```python
from build123d import *

# Parameters (mm, degrees)
SKETCH_1_R          = 12.935
EXTRUDE_1_DEPTH     = 7
SKETCH_2_R          = 14.135
EXTRUDE_2_DEPTH     = 1
SKETCH_3_R          = 11
EXTRUDE_3_DEPTH     = 7
SKETCH_4_R          = 5
CUT_EXTRUDE_1_DEPTH = 26.604617748


with BuildPart() as part:
    # 草图1 → 凸台-拉伸1 (new body)
    with BuildSketch(Plane(origin=(0, 0, 0), x_dir=(1, 0, 0), z_dir=(0, 1, 0))):
        with Locations(Location((0, 0, 0), (0, 0, 270))):
            Circle(SKETCH_1_R)
    extrude(amount=EXTRUDE_1_DEPTH)

    # 草图2 → 凸台-拉伸2 (add)
    with BuildSketch(Plane(origin=(0, 7, 0), x_dir=(1, 0, 0), z_dir=(0, 1, 0))):
        with Locations(Location((0, 0, 0), (0, 0, 270))):
            Circle(SKETCH_2_R)
    extrude_2 = extrude(amount=EXTRUDE_2_DEPTH)

    # 镜向1: 凸台-拉伸2 across plane
    add(extrude_2.mirror(Plane.ZX.offset(3.5)))

    # 草图3 → 凸台-拉伸3 (add)
    with BuildSketch(Plane(origin=(0, 8, 0), x_dir=(1, 0, 0), z_dir=(0, 1, 0))):
        with Locations(Location((0, 0, 0), (0, 0, 90))):
            Circle(SKETCH_3_R)
    extrude(amount=EXTRUDE_3_DEPTH)

    # 草图4 → 切除-拉伸1 (cut, through all)
    with BuildSketch(Plane(origin=(0, 15, 0), x_dir=(1, 0, 0), z_dir=(0, 1, 0))):
        with Locations(Location((0, 0, 0), (0, 0, 270))):
            Circle(SKETCH_4_R)
    extrude(amount=-CUT_EXTRUDE_1_DEPTH, mode=Mode.SUBTRACT)


solid = part.part
```
Model file for the job. Use its own axes, mm. A direction names the side the tool comes from. Give positions to 0.01 mm unless a question says otherwise; leave off trailing zeros. Loops run counter-clockwise (first coordinate to the right, second up) from the corner with the lowest first, then second, coordinate; pieces in that order, holes last. Notation, with made-up numbers: M 40.25,76.5 L 90.25,76.5 A24 cw 90.25,96.5 Z; hole C -25.5,9.5 d4. An arc over 180 degrees is marked long. Use one line per item in the form item = value.
Item 1: Drill centre lines: L1, parallel to X at y = 6, z = 0 (3 decimals); L2, parallel to X at y = 8.25, z = 0; L3, parallel to Y at x = 0.75, z = -12. Where is each one in solid material? Low to high.
Filled in:
L1 = -12.935 to -5, 5 to 12.935
L2 = -11 to -5, 5 to 11
L3 = -1 to 8
Item 2: Slice it at A-A on x = 0. List the corners of the cut face in (y, z) (3 decimals).
Filled in:
outline = M -1,-14.135 L 0,-14.135 L 0,-12.935 L 7,-12.935 L 7,-14.135 L 8,-14.135 L 8,-11 L 15,-11 L 15,-5 L -1,-5 Z; M -1,5 L 15,5 L 15,11 L 8,11 L 8,14.135 L 7,14.135 L 7,12.935 L 0,12.935 L 0,14.135 L -1,14.135 Z
Item 3: Which spindle directions (+Z, -Z, +X, -X, +Y, -Y) get a long thin tool onto all of the face, cutting with end or side? Do faces 4 (the cylindrical face through (14.015, -0.493, -1.84)), 5 (the cylindrical face through (10.74, 11.45, 2.38)), 6 (the cylindrical face through (-7.871, 3.451, -10.265)). Say none if no direction does.
Filled in:
face_4 = +Y, -Y
face_5 = +Y
face_6 = none
Item 4: Two-plate mould, pull along Z, no slides. Class faces 1 (the cylindrical face through (14.015, 7.493, -1.84)), 2 (the cylindrical face through (-4.88, 7.11, -1.08)), 3 (the flat face through (-4.1, 7, 12.5)): released by +Z, released by -Z, zero draft, split by the parting line, or undercut.
Filled in:
face_1 = split by the parting line
face_2 = undercut
face_3 = zero draft
Item 5: Slice it at D-D on z = -11.5. List the corners of the cut face in (x, y), and give its area (3 significant figures).
Filled in:
outline = M -8.22,-1 L 8.22,-1 L 8.22,0 L 5.92,0 L 5.92,7 L 8.22,7 L 8.22,8 L -8.22,8 L -8.22,7 L -5.92,7 L -5.92,0 L -8.22,0 Z
area = 116 mm^2
Item 6: Slice it at C-C on y = 12.5. List the corners of the cut face in (x, z), and give its area (3 significant figures).
Filled in:
outline = C 0,0 d22; hole C 0,0 d10
area = 302 mm^2
Item 7: Slice it at B-B on z = 0. List the corners of the cut face in (x, y) (3 decimals), and give its area (3 significant figures).
Filled in:
outline = M -14.135,-1 L -5,-1 L -5,15 L -11,15 L -11,8 L -14.135,8 L -14.135,7 L -12.935,7 L -12.935,0 L -14.135,0 Z; M 5,-1 L 14.135,-1 L 14.135,0 L 12.935,0 L 12.935,7 L 14.135,7 L 14.135,8 L 11,8 L 11,15 L 5,15 Z
area = 232 mm^2
Item 8: Flat gauge pins, fed straight in: pin 1 Ø2 at (x, z) = (9, 9) entering from +Y; pin 2 Ø6 at (x, y) = (-1, 12.5) entering from +Z; pin 3 Ø5 at (y, z) = (3.5, 10) entering from -X. Where does each tip first touch, or does it go through?
Filled in:
pin_1 = 8
pin_2 = 11
pin_3 = -10.54
